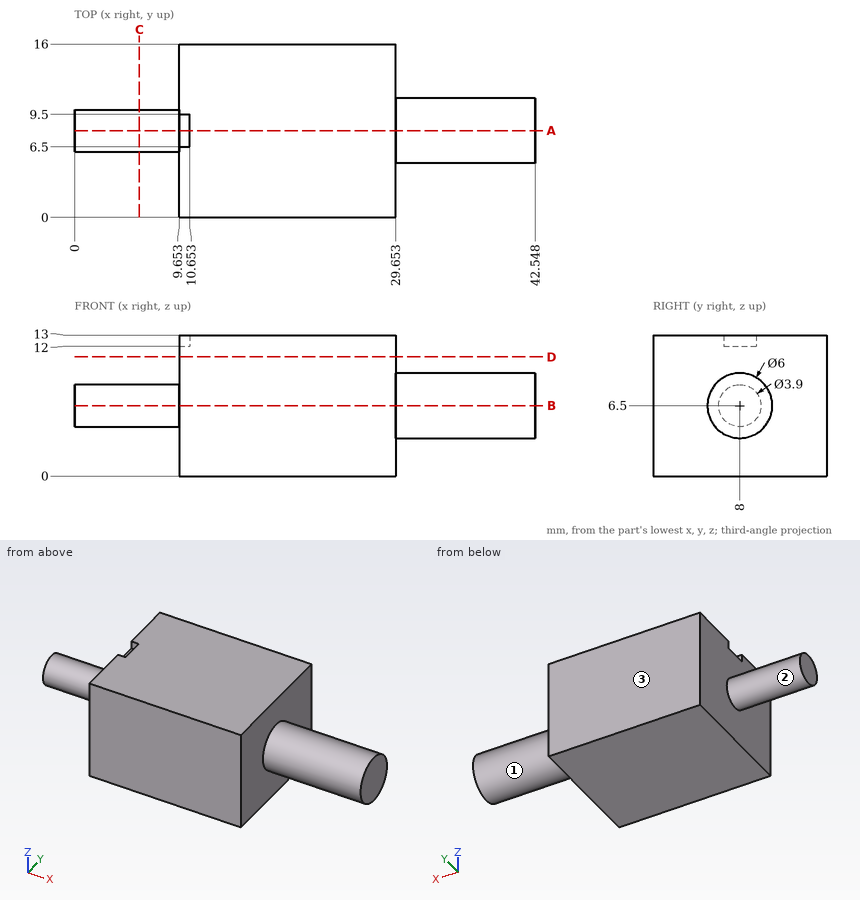
Verification items for this drawing (mm, ordinates from the low corner). A direction names the side the tool comes from. Round coordinates to 2 decimals unless told otherwise and drop trailing zeros. Order: outer loops, then holes, each group sorted by start corner. A loop starts at its lowest first (then second) coordinate and runs counter-clockwise, first axis right, second up. Notation, with made-up numbers: (9, -12) -> (19, -12) arc R29 cw to (19, 18) -> close; hole circle Ø1 at (-38, 30). An arc over 180 degrees is marked (long way). Use one line per item in the form item = value.
1. Cross-section at A-A, the plane y = 8. Enter the section's corners in (x, z).
Working result:
outline = (0, 4.55) -> (9.65, 4.55) -> (9.65, 0) -> (29.65, 0) -> (29.65, 3.5) -> (42.55, 3.5) -> (42.55, 9.5) -> (29.65, 9.5) -> (29.65, 13) -> (10.65, 13) -> (10.65, 12) -> (9.65, 12) -> (9.65, 8.45) -> (0, 8.45) -> close
2. Scan lines: line 1 along X through (y, z) = (5.25, 3.25); line 2 along X through (y, z) = (5.75, 5.5); line 3 along Y through (x, z) = (39, 6.5). Record each from-to range of solid material in increasing order. Write a range as from..to.
Working result:
line_1 = 9.65..29.65
line_2 = 9.65..42.55
line_3 = 5..11
3. Set-up check for the marked faces 1, 2 and 3: record each of +Z, -Z, +X, -X, +Y, -Y from which the full face is reachable in a straight line by a thin tool's end or side.
Working result:
face_1 = +X
face_2 = -X
face_3 = +Z, -Z, +X, -X, +Y
4. Cross-section at C-C, the plane x = 6. Enter the section's corners in (y, z).
Working result:
outline = circle Ø3.9 at (8, 6.5)
5. Cross-section at B-B, the plane z = 6.5. Enter the section's corners in (x, y), plus the area to 3 significant figures.
Working result:
outline = (0, 6.05) -> (9.65, 6.05) -> (9.65, 0) -> (29.65, 0) -> (29.65, 5) -> (42.55, 5) -> (42.55, 11) -> (29.65, 11) -> (29.65, 16) -> (9.65, 16) -> (9.65, 9.95) -> (0, 9.95) -> close
area = 435 mm^2
6. Cross-section at D-D, the plane z = 11. Enter the section's corners in (x, y), plus the area to 3 significant figures.
Working result:
outline = (9.65, 0) -> (29.65, 0) -> (29.65, 16) -> (9.65, 16) -> close
area = 320 mm^2
7. Go/stop test with flat-tipped pins: pin 1 (3 mm diameter, centred on x = 37, z = 3.5, fed in from -Y); pin 2 (1.1 mm diameter, centred on x = 10, y = 8, fed in from +Z); pin 3 (3 mm diameter, centred on x = 37, z = 7.5, fed in from +Y). Record where each tip stops, or that it passes through.
Working result:
pin_1 = 5.4
pin_2 = 12
pin_3 = 11
